For this review, take the finished solid that the model builds, in its own axes (mm). Face numbers are marked on the shaded views. Coordinates: 2 decimals unless noted, no trailing zeros. Order: outer loops, then holes, each group sorted by start corner. A loop starts at its lowest first (then second) coordinate and runs counter-clockwise, first axis right, second up.
from build123d import *

# Parameters (mm, degrees)
SKETCH1_W              = 63.5
SKETCH1_H              = 16.51
BOSS_EXTRUDE1_DEPTH    = 6.35
F_5_0MM_DOWEL_HOLE1_D  = 5
F_10_0MM_DOWEL_HOLE1_D = 10.4
F_3_0MM_DOWEL_HOLE1_D  = 3
FILLET1_R              = 5.08


with BuildPart() as part:
    # Sketch1 → Boss-Extrude1 (new body)
    with BuildSketch(Plane(origin=(0, 0, 0), x_dir=(1, 0, 0), z_dir=(0, 1, 0))):
        with Locations((31.75, 8.255)):
            Rectangle(SKETCH1_W, SKETCH1_H)
    extrude(amount=BOSS_EXTRUDE1_DEPTH)

    # Ø5.0mm Dowel Hole1 (through all)
    with Locations(Plane(origin=(0, 6.35, 0), x_dir=(1, 0, 0), z_dir=(0, 1, 0))):
        with Locations((57.15, 8.255)):
            Hole(F_5_0MM_DOWEL_HOLE1_D / 2)

    # Ø10.0mm Dowel Hole1 (through all)
    with Locations(Plane(origin=(12.7, 6.35, -8.255), x_dir=(0, 0, 1), z_dir=(0, 1, 0))):
        with Locations((0, 0)):
            Hole(F_10_0MM_DOWEL_HOLE1_D / 2)

    # Ø3.0mm Dowel Hole1 (through all)
    with Locations(Plane(origin=(0, 6.35, 0), x_dir=(1, 0, 0), z_dir=(0, 1, 0))):
        with Locations((4.699, 8.255), (20.701, 8.255)):
            Hole(F_3_0MM_DOWEL_HOLE1_D / 2)

    # Fillet1
    fillet1_edges = [part.edges().sort_by_distance(p)[0] for p in [
        (0, 3.175, -16.51),
        (63.5, 3.175, -16.51),
        (63.5, 3.175, 0),
        (0, 3.175, 0),
    ]]
    fillet(fillet1_edges, radius=FILLET1_R)


solid = part.part
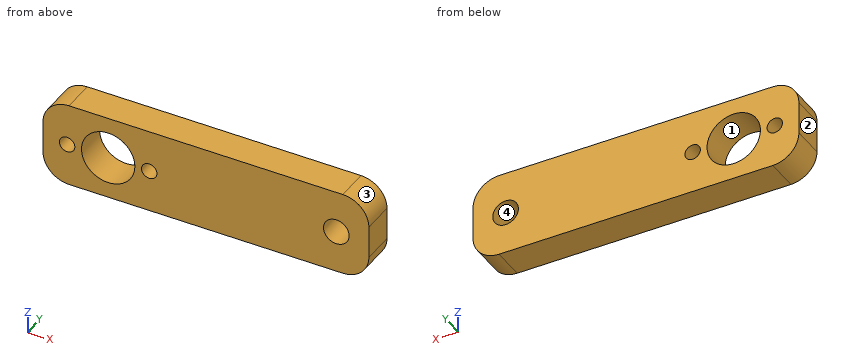
1. The part is to be moulded in two halves that separate along X. For the marked faces 1, 2, 3 and 4, say which applies: +X half, -X half, draft (parallel to the pull), parting line (faces both ways), or undercut.
Answer below:
face 1: undercut
face 2: -X half
face 3: +X half
face 4: undercut
2. To check wall thickness, follow L1, parallel to Z at x = 57.15, y = 3 (3 decimals); L2, parallel to X at y = 1.25, z = -9; L3, parallel to X at y = 4.5, z = -9.25. State the ranges of each line that lie inside material, in increasing order.
Answer below:
L1: z = -16.51 to -10.755, -5.755 to 0
L2: x = 0 to 3.4, 6 to 7.55, 17.85 to 19.4, 22 to 54.76, 59.54 to 63.5
L3: x = 0 to 3.58, 5.82 to 7.6, 17.8 to 19.58, 21.82 to 54.86, 59.44 to 63.5
3. Take a section at B-B, the plane y = 5.25. Give the boundary of the cut face in (x, z) (3 decimals), plus the area to 3 significant figures.
Answer below:
outline: (0, -11.43) arc R5.08 ccw to (5.08, -16.51) - (58.42, -16.51) arc R5.08 ccw to (63.5, -11.43) - (63.5, -5.08) arc R5.08 ccw to (58.42, 0) - (5.08, 0) arc R5.08 ccw to (0, -5.08) - close; hole circle Ø3 at (4.699, -8.255); hole circle Ø10.4 at (12.7, -8.255); hole circle Ø3 at (20.701, -8.255); hole circle Ø5 at (57.15, -8.255)
area: 908 mm2
4. Take a section at A-A, the plane x = 12.7. Give the boundary of the cut face in (y, z) (3 decimals).
Answer below:
outline: (0, -16.51) - (6.35, -16.51) - (6.35, -13.455) - (0, -13.455) - close; (0, -3.055) - (6.35, -3.055) - (6.35, 0) - (0, 0) - close
5. Take a section at C-C, the plane x = 57.15. Give the boundary of the cut face in (y, z) (3 decimals), plus the area to 3 significant figures.
Answer below:
outline: (0, -16.51) - (6.35, -16.51) - (6.35, -10.755) - (0, -10.755) - close; (0, -5.755) - (6.35, -5.755) - (6.35, 0) - (0, 0) - close
area: 73.1 mm2
6. Take a section at D-D, the plane z = -2.5. Give the boundary of the cut face in (x, y).
Answer below:
outline: (0.7, 0) - (62.8, 0) - (62.8, 6.35) - (0.7, 6.35) - close
